Design review of the part shown in the three views and the two pictorial views. Dimensions are in mm from the part's minimum x, y and z. A direction names the side the tool comes from. Give positions to 0.01 mm unless a question says otherwise; leave off trailing zeros. Loops run counter-clockwise (first coordinate to the right, second up) from the corner with the lowest first, then second, coordinate; pieces in that order, holes last. Notation, with made-up numbers: (-33.5, -16.75) -> (22.5, -16.75) arc R21 cw to (22.5, -4.75) -> close; hole circle Ø3 at (35, -31.75). An arc over 180 degrees is marked (long way). One line per question, with ' | ' between items. Start each with the question number.
(1) Wall thickness on probe 1 along Z at (x, y) = (33, 40); probe 2 along Y at (x, z) = (25, 9.75); probe 3 along Z at (x, y) = (31, 26) (3 decimals): over which ranges is each line inside the solid? List them lowest first.
(2) Consider section A-A (x = 19.5). Write out the cut boundary in (y, z) (3 decimals), and give its area (3 significant figures).
(3) Consider section C-C (y = 11). Write out the cut boundary in (x, z) (3 decimals), and give its area (3 significant figures).
(4) Consider section D-D (z = 10.75). Write out the cut boundary in (x, y) (1 decimal), and give its area (3 significant figures).
(5) Tool access review of the marked faces 1, 2 and 3: name each direction out of +Z, -Z, +X, -X, +Y, -Y from which nothing blocks a thin tool from reaching the whole face with its end or side.
(6) Insertion check: P1, Ø3, axis at x = 26, z = 7, coming from the -Y side; P2, Ø6, axis at y = 44.5, z = 7, coming from the +X side; P3, Ø9, axis at x = 28.575, y = 28.575, coming from the -Z side (3 decimals). Each pin has a flat end and moves straight along its axis. Give the tip position at first contact, or say it passes through.
(7) Consider section B-B (x = 27.5). Write out the cut boundary in (y, z) (3 decimals).
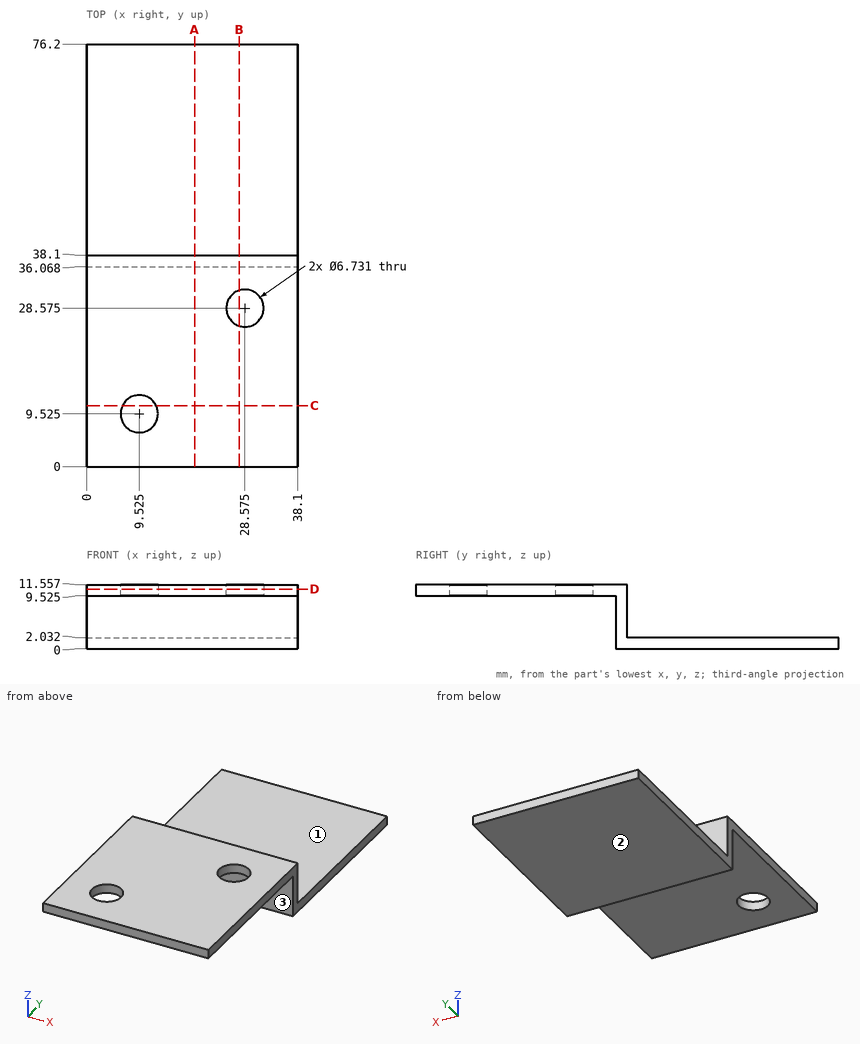
A:
1) probe 1: z = 0 to 2.03 | probe 2: y = 0 to 38.1 | probe 3: z = 9.525 to 11.557
2) outline: (0, 9.525) -> (36.068, 9.525) -> (36.068, 0) -> (76.2, 0) -> (76.2, 2.032) -> (38.1, 2.032) -> (38.1, 11.557) -> (0, 11.557) -> close | area: 174 mm^2
3) outline: (0, 9.525) -> (6.5, 9.525) -> (6.5, 11.557) -> (0, 11.557) -> close; (12.55, 9.525) -> (38.1, 9.525) -> (38.1, 11.557) -> (12.55, 11.557) -> close | area: 65.1 mm^2
4) outline: (0, 0) -> (38.1, 0) -> (38.1, 38.1) -> (0, 38.1) -> close; hole circle Ø6.7 at (9.5, 9.5); hole circle Ø6.7 at (28.6, 28.6) | area: 1,380 mm^2
5) face 1: +Z, +X, -X, +Y | face 2: -Z, +X, -X, +Y, -Y | face 3: -Z, +X, -X, -Y
6) P1: stops at y = 36.07 | P2: passes through | P3: stops at z = 9.525
7) outline: (0, 9.525) -> (25.386, 9.525) -> (25.386, 11.557) -> (0, 11.557) -> close; (31.764, 9.525) -> (36.068, 9.525) -> (36.068, 0) -> (76.2, 0) -> (76.2, 2.032) -> (38.1, 2.032) -> (38.1, 11.557) -> (31.764, 11.557) -> close
